```python
from build123d import *

# Parameters (mm, degrees)
SKETCH1_W           = 190
SKETCH1_H           = 80
SKETCH1_W_2         = 180
SKETCH1_H_2         = 70
BOSS_EXTRUDE2_DEPTH = 70
SKETCH5_W           = 185
SKETCH5_H           = 5
CUT_EXTRUDE2_DEPTH  = 75


with BuildPart() as part:
    # Sketch1 → Boss-Extrude2 (new body)
    with BuildSketch(Plane(origin=(0, 0, 0), x_dir=(1, 0, 0), z_dir=(0, 1, 0))):
        with Locations((95, 40)):
            Rectangle(SKETCH1_W, SKETCH1_H)
        with Locations((95, 40)):
            Rectangle(SKETCH1_W_2, SKETCH1_H_2, mode=Mode.SUBTRACT)
    extrude(amount=BOSS_EXTRUDE2_DEPTH)

    # Sketch5 → Cut-Extrude2 (cut)
    with BuildSketch(Plane(origin=(0, 0, -80), x_dir=(-1, 0, 0), z_dir=(0, 0, -1))):
        with Locations((-95, 62.5)):
            Rectangle(SKETCH5_W, SKETCH5_H)
    extrude(amount=-CUT_EXTRUDE2_DEPTH, mode=Mode.SUBTRACT)


solid = part.part
```
CAD build for the part. Positions are in the model's coordinates, mm. A direction names the side the tool comes from. Round coordinates to 2 decimals unless told otherwise and drop trailing zeros. Order: outer loops, then holes, each group sorted by start corner. A loop starts at its lowest first (then second) coordinate and runs counter-clockwise, first axis right, second up.
Q1. Wall check: L1, parallel to X at y = 46.5, z = -58.5; L2, parallel to Z at x = 82, y = 58.5; L3, parallel to X at y = 61, z = -31. Give the ranges that are in metal, low to high.
Q2. Slice it at B-B (z = -7.5). Write the cut outline in (x, y).
Q3. Two-plate mould, pull along X, no slides. Class faces 1 (the flat face through (94, 35, -5)), 2 (the flat face through (0, 35, -39)), 3 (the flat face through (94, 35, 0)), 4 (the flat face through (95, 60, -76)): pulls with the +X half, pulls with the -X half, needs draft (parallel to the pull), parting line crosses it, or undercut.
Q4. Slice it at C-C (y = 39.5). Write the cut outline in (x, z), and give its area (3 significant figures).
Q5. Which spindle directions (+Z, -Z, +X, -X, +Y, -Y) get a long thin tool onto all of the face, cutting with end or side? Do faces 5 (the flat face through (87.5, 70, -4.6)), 6 (the flat face through (185, 30, -40)), 7 (the flat face through (95, 65, -76)). Say none if no direction does.
Q6. Slice it at A-A (x = 24.5). Write the cut outline in (y, z), and give its area (3 significant figures).
Q7. Slice it at D-D (y = 63). Write the cut outline in (x, z).
Results below:
1. L1: x = 0 to 5, 185 to 190
1. L2: z = -80 to -75, -5 to 0
1. L3: x = 0 to 2.5, 187.5 to 190
2. outline: (0, 0) - (5, 0) - (5, 60) - (2.5, 60) - (2.5, 65) - (5, 65) - (5, 70) - (0, 70) - close; (185, 0) - (190, 0) - (190, 70) - (185, 70) - (185, 65) - (187.5, 65) - (187.5, 60) - (185, 60) - close
3. face 1: undercut
3. face 2: pulls with the -X half
3. face 3: needs draft
3. face 4: undercut
4. outline: (0, -80) - (190, -80) - (190, 0) - (0, 0) - close; hole (5, -75) - (185, -75) - (185, -5) - (5, -5) - close
4. area: 2,600 mm2
5. face 5: +Z, -Z, +X, -X, +Y
5. face 6: +Y, -Y
5. face 7: -Z
6. outline: (0, -80) - (60, -80) - (60, -75) - (0, -75) - close; (0, -5) - (70, -5) - (70, 0) - (0, 0) - close; (65, -80) - (70, -80) - (70, -75) - (65, -75) - close
6. area: 675 mm2
7. outline: (0, -80) - (2.5, -80) - (2.5, -5) - (187.5, -5) - (187.5, -80) - (190, -80) - (190, 0) - (0, 0) - close
